Build history of the part. All positions in model axes, mm. A direction names the side the tool comes from. Round coordinates to 2 decimals unless told otherwise and drop trailing zeros. Write each loop counter-clockwise with the first axis right and the second up, starting at its lowest first coordinate (ties: lowest second). Pieces come first, ordered by that corner, then holes. Notation, with made-up numbers: M -5.75,-5.5 L 2.25,-5.5 A3 cw 2.25,-1.5 Z; hole C 87,48 d6. An arc over 180 degrees is marked long. Use a Markdown table: item, result.
from build123d import *

# Parameters (mm, degrees)
F0_W     = 77.5562152267
F0_H     = 114.8829683661
F1_DEPTH = 12.5
F2_T     = -2.54
F3_R     = 5.08
F4_R     = 5.08


with BuildPart() as f1:
    # F0 (on Front) → F1 (new body, symmetric)
    with BuildSketch(Plane.XZ):
        Rectangle(F0_W, F0_H)
    extrude(amount=F1_DEPTH, both=True)

    # F2
    f2_openings = [f1.faces().sort_by_distance(p)[0] for p in [
        (0, -12.5, 0),
    ]]
    offset(amount=F2_T, openings=f2_openings)

    # F3
    f3_edges = [f1.edges().sort_by_distance(p)[0] for p in [
        (0, 9.96, -54.901484),
        (36.238108, 9.96, 0),
        (0, 9.96, 54.901484),
        (-36.238108, 9.96, 0),
    ]]
    fillet(f3_edges, radius=F3_R)

    # F4
    f4_edges = [f1.edges().sort_by_distance(p)[0] for p in [
        (-38.778108, 0, 57.441484),
        (38.778108, 0, 57.441484),
        (38.778108, 0, -57.441484),
        (-38.778108, 0, -57.441484),
    ]]
    fillet(f4_edges, radius=F4_R)


solid = f1.part
Q1. Cut at A-A on y = -7.5. Give the cut face in (x, z), and give its area (3 significant figures).
Response values:
| item | result |
|---|---|
| outline | M -38.78,-52.36 A5.08 ccw -33.7,-57.44 L 33.7,-57.44 A5.08 ccw 38.78,-52.36 L 38.78,52.36 A5.08 ccw 33.7,57.44 L -33.7,57.44 A5.08 ccw -38.78,52.36 Z; hole M -36.24,-54.9 L 36.24,-54.9 L 36.24,54.9 L -36.24,54.9 Z |
| area | 930 mm2 |
Q2. Drill centre lines: L1, parallel to Z at x = 23.5, y = -8.25; L2, parallel to X at y = -7.25, z = 10.5; L3, parallel to Y at x = -18, z = 41.5. Where is each one in solid material? Low to high.
Response values:
| item | result |
|---|---|
| L1 | z = -57.44 to -54.9, 54.9 to 57.44 |
| L2 | x = -38.78 to -36.24, 36.24 to 38.78 |
| L3 | y = 9.96 to 12.5 |
Q3. Drop a flat-ended pin along its axis: P1, Ø6, axis at x = -15, z = -13.5, coming from the -Y side. Give the stop position or say it passes through.
Response values:
| item | result |
|---|---|
| P1 | stops at y = 9.96 |
Q4. Two-plate mould, pull along X, no slides. Class faces 3 (the cylindrical face through (-37.329, 0.175, 55.914)), 4 (the flat face through (38.778, 0, -1)), 5 (the cylindrical face through (34.79, 8.43, -0.77)): +X half, -X half, draft (parallel to the pull), parting line (faces both ways), or undercut.
Response values:
| item | result |
|---|---|
| face 3 | -X half |
| face 4 | +X half |
| face 5 | undercut |
Q5. Cut at B-B on x = -5.5. Give the cut face in (y, z).
Response values:
| item | result |
|---|---|
| outline | M -12.5,-57.44 L 12.5,-57.44 L 12.5,57.44 L -12.5,57.44 L -12.5,54.9 L 4.88,54.9 A5.08 cw 9.96,49.82 L 9.96,-49.82 A5.08 cw 4.88,-54.9 L -12.5,-54.9 Z |
Q6. Which spindle directions (+Z, -Z, +X, -X, +Y, -Y) get a long thin tool onto all of the face, cutting with end or side? Do faces 1 (the flat face through (-1, 12.5, 1)), 2 (the flat face through (-1, -4, 54.901)). Say none if no direction does.
Response values:
| item | result |
|---|---|
| face 1 | +Z, -Z, +X, -X, +Y |
| face 2 | -Y |
Q7. Cut at C-C on z = -11. Give the cut face in (x, y).
Response values:
| item | result |
|---|---|
| outline | M -38.78,-12.5 L -36.24,-12.5 L -36.24,4.88 A5.08 cw -31.16,9.96 L 31.16,9.96 A5.08 cw 36.24,4.88 L 36.24,-12.5 L 38.78,-12.5 L 38.78,12.5 L -38.78,12.5 Z |
